The listing builds one solid part. Answer for the finished solid, in the listing's coordinates (mm). A direction names the side the tool comes from. Round coordinates to 2 decimals unless told otherwise and drop trailing zeros. Write each loop counter-clockwise with the first axis right and the second up, starting at its lowest first coordinate (ties: lowest second). Pieces come first, ordered by that corner, then holes.
(1) A cutting plane is placed at B-B, the plane z = -32.5. Give the vertices of the cut face in (x, y), and give its area (3 significant figures).
(2) The mould has two halves that part along Z. Classify faces 4 (the face through (2, 2, -25)), 5 (the face through (2, 40, -63)), 6 (the face through (2, 2, -10)), 7 (the face through (2, 2, -55)): +Z half, -Z half, draft (parallel to the pull), parting line (faces both ways), or undercut.
(3) A cutting plane is placed at A-A, the plane y = 32.5. Give the vertices of the cut face in (x, z), and give its area (3 significant figures).
(4) A cutting plane is placed at C-C, the plane y = 58.5. Give the vertices of the cut face in (x, z), and give its area (3 significant figures).
(5) Find the intervals of material crossed by probe 1 along Y at (x, z) = (1.75, -32.5); probe 2 along Z at (x, y) = (1.3, 3); probe 3 along Y at (x, z) = (1.05, -39), in increasing order.
(6) Each of these flat-tipped pins is pushed along its axis until it touches: pin 1 Ø2 at (x, y) = (2.5, 6.5) entering from +Z; pin 2 Ø2 at (x, z) = (2.5, -63.5) entering from +Y; pin 3 Ø2 at (x, y) = (3, 23.5) entering from +Z; pin 4 Ø2 at (x, y) = (1.5, 7) entering from -Z. Where does it stop, or does it pass through?
(7) For faces 1 (the face through (2, 4, -7)), 2 (the face through (2, 4, -58)), 3 (the face through (2, 40, -2)), determine the directions among +Z, -Z, +X, -X, +Y, -Y from which every point of the face is accessible in a straight line to the end or side of a thin tool.
from build123d import *

# Parameters (mm, degrees)
SKETCH1_W           = 65
SKETCH1_H           = 65
BOSS_EXTRUDE1_DEPTH = 4
SKETCH2_R           = 5
CUT_EXTRUDE1_DEPTH  = 4
SKETCH3_W           = 10
SKETCH3_H           = 4
SKETCH3_W_2         = 15
CUT_EXTRUDE2_DEPTH  = 4
SKETCH5_W           = 4
SKETCH5_H           = 6
SKETCH5_H_2         = 15
CUT_EXTRUDE3_DEPTH  = 4


with BuildPart() as part:
    # Sketch1 → Boss-Extrude1 (new body)
    with BuildSketch(Plane(origin=(0, 0, 0), x_dir=(0, 0, -1), z_dir=(1, 0, 0))):
        with Locations((32.5, 32.5)):
            Rectangle(SKETCH1_W, SKETCH1_H)
    extrude(amount=BOSS_EXTRUDE1_DEPTH)

    # Sketch2 → Cut-Extrude1 (cut)
    with BuildSketch(Plane(origin=(4, 0, 0), x_dir=(0, 0, -1), z_dir=(1, 0, 0))):
        with Locations((32.5, 32.5)):
            Circle(SKETCH2_R)
    extrude(amount=-CUT_EXTRUDE1_DEPTH, mode=Mode.SUBTRACT)

    # Sketch3 → Cut-Extrude2 (cut)
    with BuildSketch(Plane(origin=(4, 0, 0), x_dir=(0, 0, -1), z_dir=(1, 0, 0))):
        with Locations((5, 63)):
            Rectangle(SKETCH3_W, SKETCH3_H)
        with Locations((32.5, 63)):
            Rectangle(SKETCH3_W_2, SKETCH3_H)
        with Locations((60, 63)):
            Rectangle(SKETCH3_W, SKETCH3_H)
        with Locations((60, 2)):
            Rectangle(SKETCH3_W, SKETCH3_H)
        with Locations((32.5, 2)):
            Rectangle(SKETCH3_W_2, SKETCH3_H)
        with Locations((5, 2)):
            Rectangle(SKETCH3_W, SKETCH3_H)
    extrude(amount=-CUT_EXTRUDE2_DEPTH, mode=Mode.SUBTRACT)

    # Sketch5 → Cut-Extrude3 (cut)
    with BuildSketch(Plane(origin=(4, 0, 0), x_dir=(0, 0, -1), z_dir=(1, 0, 0))):
        with Locations((2, 58)):
            Rectangle(SKETCH5_W, SKETCH5_H)
        with Locations((2, 32.5)):
            Rectangle(SKETCH5_W, SKETCH5_H_2)
        with Locations((2, 7)):
            Rectangle(SKETCH5_W, SKETCH5_H)
        with Locations((63, 7)):
            Rectangle(SKETCH5_W, SKETCH5_H)
        with Locations((63, 32.5)):
            Rectangle(SKETCH5_W, SKETCH5_H_2)
        with Locations((63, 58)):
            Rectangle(SKETCH5_W, SKETCH5_H)
    extrude(amount=-CUT_EXTRUDE3_DEPTH, mode=Mode.SUBTRACT)


solid = part.part
Solutions:
1. outline: (0, 4) - (4, 4) - (4, 27.5) - (0, 27.5) - close; (0, 37.5) - (4, 37.5) - (4, 61) - (0, 61) - close
1. area: 188 mm2
2. face 4: undercut
2. face 5: draft
2. face 6: +Z half
2. face 7: -Z half
3. outline: (0, -61) - (4, -61) - (4, -37.5) - (0, -37.5) - close; (0, -27.5) - (4, -27.5) - (4, -4) - (0, -4) - close
3. area: 188 mm2
4. outline: (0, -61) - (4, -61) - (4, -4) - (0, -4) - close
4. area: 228 mm2
5. probe 1: y = 4 to 27.5, 37.5 to 61
5. probe 2: z = -55 to -40, -25 to -10
5. probe 3: y = 4 to 61
6. pin 1: stops at z = -4
6. pin 2: stops at y = 55
6. pin 3: stops at z = 0
6. pin 4: stops at z = -61
7. face 1: +Z, +X, -X, -Y
7. face 2: -Z, +X, -X, -Y
7. face 3: +Z, +X, -X
